```python
from build123d import *

# Parameters (mm, degrees)
F0_W     = 120
F0_H     = 65
F1_DEPTH = 30
F2_R     = 10
F3_W     = 158.2465842366
F3_H     = 88.3002289823
F4_DEPTH = 60
F5_T     = 1


with BuildPart() as f1:
    # F0 (on Front) → F1 (new body, symmetric)
    with BuildSketch(Plane.XZ):
        with Locations((-0.1071500592, 0.0989875504)):
            Rectangle(F0_W, F0_H)
    extrude(amount=F1_DEPTH, both=True)

    # F2
    f2_edges = [f1.edges().sort_by_distance(p)[0] for p in [
        (-0.10715, -30, -32.401012),
        (59.89285, 0, -32.401012),
        (-0.10715, 30, -32.401012),
        (-60.10715, 0, -32.401012),
        (-0.10715, -30, 32.598988),
        (59.89285, 0, 32.598988),
        (-60.10715, 0, 32.598988),
        (-0.10715, 30, 32.598988),
        (-60.10715, 30, 0.098988),
        (-60.10715, -30, 0.098988),
        (59.89285, -30, 0.098988),
        (59.89285, 30, 0.098988),
    ]]
    fillet(f2_edges, radius=F2_R)

    # F3 (on face) → F4 (cut)
    with BuildSketch(Plane.XZ.offset(30)):
        with Locations((1.5532188118, 44.2491020416)):
            Rectangle(F3_W, F3_H)
    extrude(amount=-F4_DEPTH, mode=Mode.SUBTRACT)

    # F5
    f5_openings = [f1.faces().sort_by_distance(p)[0] for p in [
        (-0.10715, 0, 0.098988),
    ]]
    offset(amount=F5_T, openings=f5_openings)

    # F6: F1 across face


with BuildPart() as f1_1:
    add(f1.part)
    add(f1.part.mirror(Plane(origin=(-0.1071500592, 0, 0.0989875504), x_dir=(1, 0, 0), z_dir=(0, 0, 1))))


solid = f1_1.part
```
Geometry: final body of the model. Coordinates: model frame, mm. A direction names the side the tool comes from. Coordinates: 2 decimals unless noted, no trailing zeros. Order: outer loops, then holes, each group sorted by start corner. A loop starts at its lowest first (then second) coordinate and runs counter-clockwise, first axis right, second up. Notation, with made-up numbers: (32.5, 42.5) - (70.5, 42.5) arc R24 cw to (70.5, 63.5) - close; hole circle Ø1 at (18, 55). An arc over 180 degrees is marked (long way). Return JSON: item names as keys, results as strings. Group by question number.
1. Set-up query: faces 5 (the face through (-57.26, -0.28, 29.59)), 6 (the face through (-57.97, -0.28, -30.093)). Return all of +Z, -Z, +X, -X, +Y, -Y with unobstructed straight access to the full face (end or side cutting, diameter ignored); none if empty.
2. Material intervals for line 1 along X through (y, z) = (-7, 9); line 2 along Z through (x, y) = (46.5, 18.5); line 3 along Y through (x, z) = (8, 14.5), sorted ascending. Write a range as [from, to].
3. Cut plane B-B (x = -16.5). Output: boundary loops of the cut face in (y, z).
4. Pull-direction query (Z, two-part tool) for faces 1 (the face through (0.59, 27.15, 29.59)), 2 (the face through (0.593, 27.863, 30.291)), 3 (the face through (57.041, 26.993, -0.216)), 4 (the face through (-57.97, -27.69, -0.22)); classes: pulls with the +Z half, pulls with the -Z half, needs draft (parallel to the pull), parting line crosses it, or undercut.
5. Cut plane A-A (y = 3.5). Output: boundary loops of the cut face in (x, z), plus the area to 3 significant figures.
Resolved:
{
 "1": {"face 5": "none", "face 6": "-Z, -X, +Y, -Y"},
 "2": {"line 1": "x = [-61.11, -60.11], [59.89, 60.89]", "line 2": "z = [-33.4, -32.4], [32.6, 33.6]", "line 3": "y = [-31, -30], [30, 31]"},
 "3": {"outline": "(-31, -22.4) arc R11 ccw to (-20, -33.4) - (20, -33.4) arc R11 ccw to (31, -22.4) - (31, 22.6) arc R11 ccw to (20, 33.6) - (-20, 33.6) arc R11 ccw to (-31, 22.6) - close; hole (-30, -22.4) arc R10 ccw to (-20, -32.4) - (20, -32.4) arc R10 ccw to (30, -22.4) - (30, 22.6) arc R10 ccw to (20, 32.6) - (-20, 32.6) arc R10 ccw to (-30, 22.6) - close"},
 "4": {"face 1": "undercut", "face 2": "pulls with the +Z half", "face 3": "undercut", "face 4": "needs draft"},
 "5": {"outline": "(-61.11, -22.4) arc R11 ccw to (-50.11, -33.4) - (49.89, -33.4) arc R11 ccw to (60.89, -22.4) - (60.89, 22.6) arc R11 ccw to (49.89, 33.6) - (-50.11, 33.6) arc R11 ccw to (-61.11, 22.6) - close; hole (-60.11, -22.4) arc R10 ccw to (-50.11, -32.4) - (49.89, -32.4) arc R10 ccw to (59.89, -22.4) - (59.89, 22.6) arc R10 ccw to (49.89, 32.6) - (-50.11, 32.6) arc R10 ccw to (-60.11, 22.6) - close", "area": "356 mm²"}
}
